```python
from build123d import *

# Parameters (mm, degrees)
F0_W        = 35
F0_H        = 20
F1_DEPTH    = 45
F2_W        = 29
F2_H        = 14
F3_DEPTH    = 40
F4_T1_DEPTH = 45
F4_T3_DEPTH = 60


# Not quite as in the source:
# - a fillet or chamfer that OpenCascade refuses, or shapes differently, is made with other operations: its cross-section is extruded or revolved along the edge and cut away or added
# - a feature names something its author has since deleted; it is built from what else it names


with BuildPart() as f1:
    # F0 (on Top) → F1 (new body)
    with BuildSketch(Plane.XY):
        Rectangle(F0_W, F0_H)
    extrude(amount=F1_DEPTH)

    # F2 (on face) → F3 (cut)
    with BuildSketch(Plane.XY.offset(45)):
        Rectangle(F2_W, F2_H)
    extrude(amount=-F3_DEPTH, mode=Mode.SUBTRACT)

    # F4: fillet of radius 5 on 4 edges, made by hand

    # F4_s2 → F4_t1 (cut)
    with BuildSketch(Plane.XZ.offset(-22.5)):
        with BuildLine():
            ThreePointArc((17.5, 40), (16.0355339059, 43.5355339059), (12.5, 45))
            Line((12.5, 45), (17.5, 45))
            Line((17.5, 45), (17.5, 40))
        make_face()
        with BuildLine():
            ThreePointArc((-17.5, 40), (-16.0355339059, 43.5355339059), (-12.5, 45))
            Line((-12.5, 45), (-17.5, 45))
            Line((-17.5, 45), (-17.5, 40))
        make_face()
    extrude(amount=F4_T1_DEPTH, mode=Mode.SUBTRACT)

    # F4_s4 → F4_t3 (cut)
    with BuildSketch(Plane.YZ.offset(-30)):
        with BuildLine():
            ThreePointArc((-5, 45), (-8.5355339059, 43.5355339059), (-10, 40))
            Line((-10, 40), (-10, 45))
            Line((-10, 45), (-5, 45))
        make_face()
        with BuildLine():
            ThreePointArc((10, 40), (8.5355339059, 43.5355339059), (5, 45))
            Line((5, 45), (10, 45))
            Line((10, 45), (10, 40))
        make_face()
    extrude(amount=F4_T3_DEPTH, mode=Mode.SUBTRACT)


solid = f1.part
```
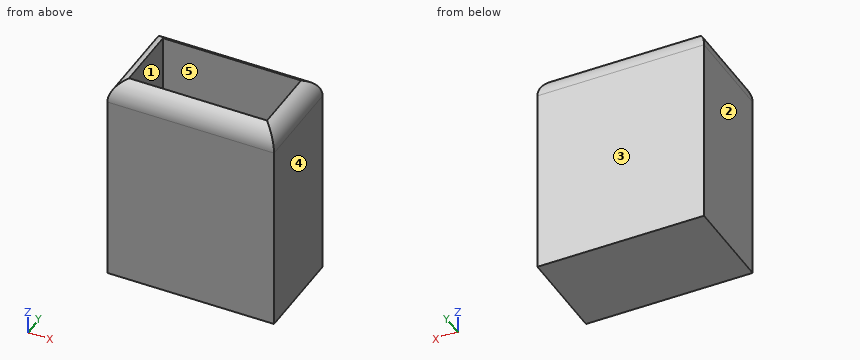
Source: CAD feature listing. Evaluate the final solid. Frame: model axes, mm. Face numbers are marked on the shaded views. A direction names the side the tool comes from. Give positions to 0.01 mm unless a question says otherwise; leave off trailing zeros. Order: outer loops, then holes, each group sorted by start corner. A loop starts at its lowest first (then second) coordinate and runs counter-clockwise, first axis right, second up.
(1) Contact query for flat-ended pins moving along their axis: P1, Ø1, axis at x = 4, y = 7, coming from the -Z side; P2, Ø4, axis at x = -4, y = -1, coming from the +Z side. Output: stop coordinate, or through.
(2) Section query A-A (z = 39). Return the cut outline in (x, y).
(3) Section query B-B (x = -5). Return the cut outline in (y, z).
(4) Section query C-C (y = -4). Return the cut outline in (x, z).
(5) Access query for the marked faces 1 and 2. Directions: +Z, -Z, +X, -X, +Y, -Y. A direction counts if a zero-diameter tool reaches every point of the face in a straight line with its end or side. Return the directions, or none.
(6) Material intervals for line 1 along Y through (x, z) = (3, 23); line 2 along X through (y, z) = (-0.5, 29.5); line 3 along Z through (x, y) = (-5.5, 2.5), sorted ascending.
(7) Pull-direction query (Y, two-part tool) for the marked faces 3, 4 and 5; classes: +Y half, -Y half, draft (parallel to the pull), parting line (faces both ways), or undercut.
Outcome:
1. P1: stops at z = 0
1. P2: stops at z = 5
2. outline: (-17.5, -10) - (17.5, -10) - (17.5, 10) - (-17.5, 10) - close; hole (-14.5, -7) - (14.5, -7) - (14.5, 7) - (-14.5, 7) - close
3. outline: (-10, 0) - (10, 0) - (10, 40) arc R5 ccw to (7, 44.58) - (7, 5) - (-7, 5) - (-7, 44.58) arc R5 ccw to (-10, 40) - close
4. outline: (-17.5, 0) - (17.5, 0) - (17.5, 40) arc R5 ccw to (14.5, 44.58) - (14.5, 5) - (-14.5, 5) - (-14.5, 44.58) arc R5 ccw to (-17.5, 40) - close
5. face 1: +Z
5. face 2: +Z, -Z, -X, +Y, -Y
6. line 1: y = -10 to -7, 7 to 10
6. line 2: x = -17.5 to -14.5, 14.5 to 17.5
6. line 3: z = 0 to 5
7. face 3: +Y half
7. face 4: draft
7. face 5: undercut
